Answer from the drawing. Dimensions are ordinates in mm from the lowest x, y and z of the part. A direction names the side the tool comes from. Round coordinates to 2 decimals unless told otherwise and drop trailing zeros. Order: outer loops, then holes, each group sorted by start corner. A loop starts at its lowest first (then second) coordinate and runs counter-clockwise, first axis right, second up. Notation, with made-up numbers: (22, -4) -> (72, -4) arc R21 cw to (72, 7) -> close; hole circle Ø9 at (60, -39.5). An arc over 180 degrees is marked (long way). Use a Markdown table: item, result. Add a question column.
1. Section B-B, the plane x = 19.25 is taken. Give the vertices of the cut face in (y, z).
2. Given pin 1 (1.9 mm diameter, centred on x = 13.5, z = 10.5, fed in from -Y), flat-ended and moving along its own axis, determine where the tip first touches the part or whether it passes through.
3. Consider L1, parallel to Z at x = 3.25, y = 3.5; L2, parallel to Z at x = 8.5, y = 2.25; L3, parallel to Z at x = 22, y = 1.25. Determine where each line is inside the solid, lowest interval first. Write a range as [from, to].
4. Section D-D, the plane x = 4 is taken. Give the vertices of the cut face in (y, z).
5. For the marked faces 1 and 2, determine the directions among +Z, -Z, +X, -X, +Y, -Y from which every point of the face is accessible in a straight line to the end or side of a thin tool.
6. The mould has two halves that part along Z. Classify the marked faces 3, 4 and 5: +Z half, -Z half, draft (parallel to the pull), parting line (faces both ways), or undercut.
7. Section A-A, the plane y = 0.5 is taken. Give the number of separate pieces and of enclosed holes in the cut face, then the cut area to 3 significant figures.
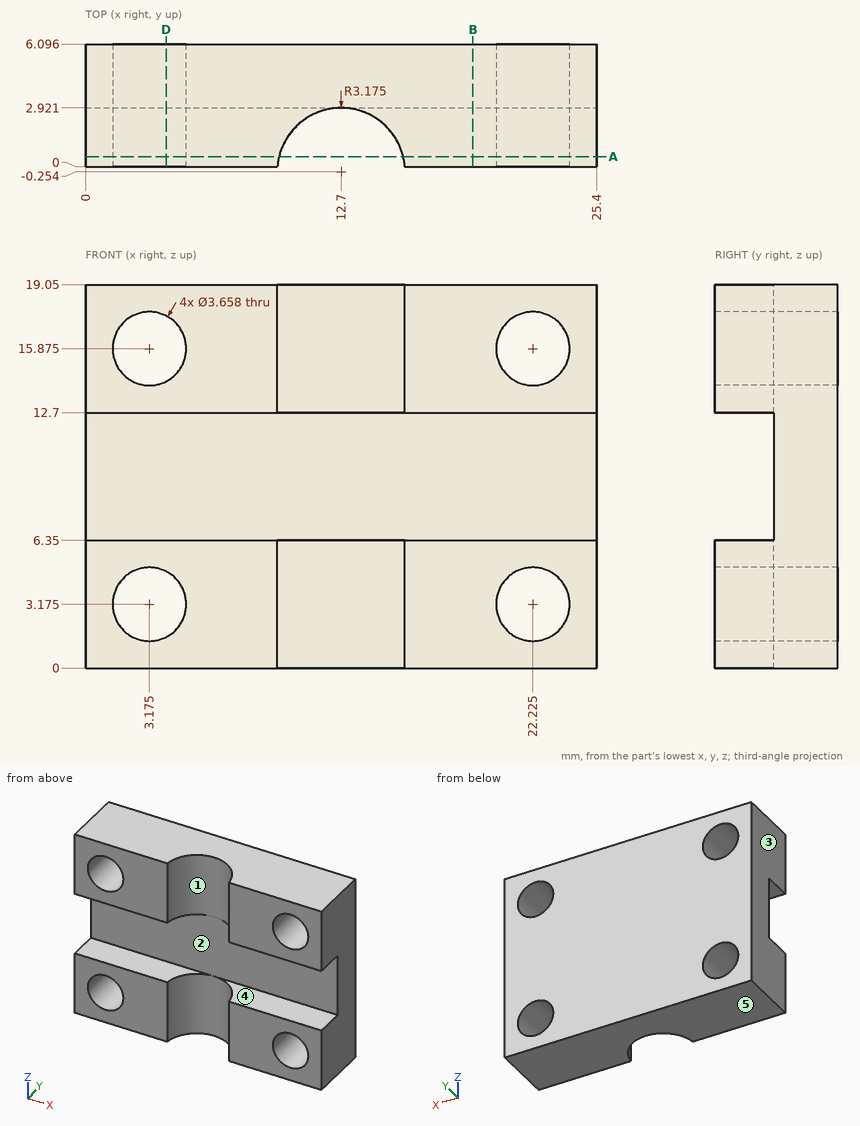
Verdict:
| question | item | result |
|---|---|---|
| 1 | outline | (0, 0) -> (6.1, 0) -> (6.1, 19.05) -> (0, 19.05) -> (0, 12.7) -> (2.92, 12.7) -> (2.92, 6.35) -> (0, 6.35) -> close |
| 2 | pin 1 | stops at y = 2.92 |
| 3 | L1 | z = [0, 1.35], [5, 14.05], [17.7, 19.05] |
| 3 | L2 | z = [0, 6.35], [12.7, 19.05] |
| 3 | L3 | z = [0, 1.36], [4.99, 6.35], [12.7, 14.06], [17.69, 19.05] |
| 4 | outline | (0, 0) -> (6.1, 0) -> (6.1, 1.54) -> (0, 1.54) -> close; (0, 4.81) -> (6.1, 4.81) -> (6.1, 14.24) -> (0, 14.24) -> (0, 12.7) -> (2.92, 12.7) -> (2.92, 6.35) -> (0, 6.35) -> close; (0, 17.51) -> (6.1, 17.51) -> (6.1, 19.05) -> (0, 19.05) -> close |
| 5 | face 1 | +Z, -Z, -Y |
| 5 | face 2 | +X, -X, -Y |
| 6 | face 3 | draft |
| 6 | face 4 | undercut |
| 6 | face 5 | -Z half |
| 7 | separate pieces | 4 |
| 7 | enclosed holes | 4 |
| 7 | area | 202 mm2 |
